```python
from build123d import *

# Parameters (mm, degrees)
SKETCH_W             = 55.4
SKETCH_H             = 49
PAD_DEPTH            = 24.5
SKETCH001_W          = 20.2
SKETCH001_H          = 39
POCKET_DEPTH         = 49
SKETCH002_W          = 20.2
SKETCH002_H          = 39
POCKET001_DEPTH      = 24.501
POCKET001_DEPTH_BACK = 24.501
SKETCH003_R          = 12.5
POCKET002_DEPTH      = 27.701
POCKET002_DEPTH_BACK = 27.701
CHAMFER_SIZE         = 1


with BuildPart() as part:
    # Sketch → Pad (new body, symmetric)
    with BuildSketch(Plane.XY):
        Rectangle(SKETCH_W, SKETCH_H)
    extrude(amount=PAD_DEPTH, both=True)

    # Sketch001 → Pocket (cut)
    with BuildSketch(Plane.XY.offset(29.5)):
        with Locations((12.6, 0)):
            Rectangle(SKETCH001_W, SKETCH001_H)
    extrude(amount=-POCKET_DEPTH, mode=Mode.SUBTRACT)

    # Sketch002 → Pocket001 (cut, two sides)
    with BuildSketch(Plane.XZ) as pocket001_sk:
        with Locations((-12.6, 0)):
            Rectangle(SKETCH002_W, SKETCH002_H)
    extrude(amount=-POCKET001_DEPTH, mode=Mode.SUBTRACT)
    extrude(pocket001_sk.sketch, amount=POCKET001_DEPTH_BACK, mode=Mode.SUBTRACT)

    # Sketch003 → Pocket002 (cut, two sides)
    with BuildSketch(Plane.YZ) as pocket002_sk:
        Circle(SKETCH003_R)
    extrude(amount=-POCKET002_DEPTH, mode=Mode.SUBTRACT)
    extrude(pocket002_sk.sketch, amount=POCKET002_DEPTH_BACK, mode=Mode.SUBTRACT)

    # Chamfer
    chamfer_edges = [part.edges().sort_by_distance(p)[0] for p in [
        (0, -24.5, 24.5),
        (-27.7, -24.5, 0),
        (0, -24.5, -24.5),
        (-12.6, -24.5, -19.5),
        (-22.7, -24.5, 0),
        (-12.6, -24.5, 19.5),
        (-2.5, -24.5, 0),
        (27.7, -24.5, 0),
        (27.7, 0, 24.5),
        (27.7, -12.5, 0),
        (27.7, 0, -24.5),
        (27.7, 24.5, 0),
        (22.7, 0, 24.5),
        (12.6, -19.5, 24.5),
        (2.5, 0, 24.5),
        (12.6, 19.5, 24.5),
        (-27.7, 0, 24.5),
        (0, 24.5, 24.5),
        (2.5, -12.5, 0),
        (22.7, -12.5, 0),
        (0, 24.5, -24.5),
        (-2.5, 24.5, 0),
        (-12.6, 24.5, -19.5),
        (-22.7, 24.5, 0),
        (-12.6, 24.5, 19.5),
        (-27.7, 24.5, 0),
        (-27.7, 0, -24.5),
        (-27.7, -12.5, 0),
        (-22.7, -12.5, 0),
        (-2.5, -12.5, 0),
    ]]
    chamfer(chamfer_edges, length=CHAMFER_SIZE)


solid = part.part
```
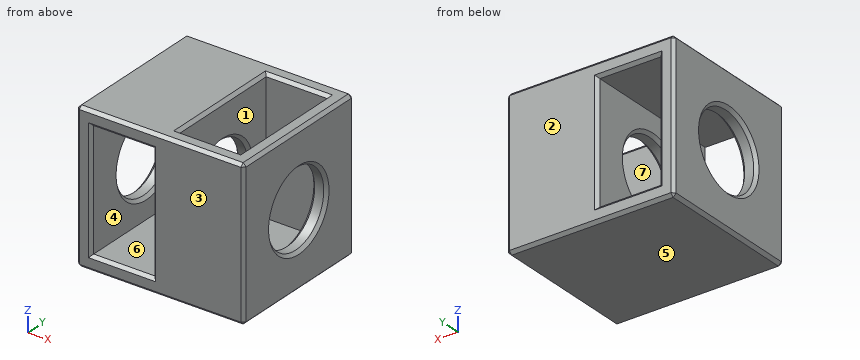
Geometry: final body of the model. Coordinates: model frame, mm. Face numbers are marked on the shaded views. A direction names the side the tool comes from. Coordinates: 2 decimals unless noted, no trailing zeros. Write each loop counter-clockwise with the first axis right and the second up, starting at its lowest first coordinate (ties: lowest second). Pieces come first, ordered by that corner, then holes. Notation, with made-up numbers: M 38,25.25 L 64,25.25 A16 ccw 64,36.25 Z; hole C -30,33.25 d6. An arc over 180 degrees is marked long. Use CSV: the item, a comma, the result in double quotes. Start each with the question number.
1. Cut plane A-A on y = -15.5. Return the cut outline in (x, z), plus the area to 4 significant figures.
2. Cut plane C-C on x = 9.5. Return the cut outline in (y, z).
3. Cut plane B-B on x = -11. Return the cut outline in (y, z), plus the area to 3 significant figures.
4. Ray query, probe 1 along X at (y, z) = (12, 9); probe 2 along Y at (x, z) = (0.5, 0); probe 3 along Y at (x, z) = (16.5, 13). Return the intervals inside material, ascending.
5. Mould query, pull axis Y, two halves, no side actions, for the marked faces 1, 2, 3 and 4. Classes: pulls with the +Y half, pulls with the -Y half, needs draft (parallel to the pull), parting line crosses it, or undercut.
6. Reachability of the marked faces 5, 6 and 7 from +Z, -Z, +X, -X, +Y, -Y: full face, straight path, thin tool, end or side. Return the list, or none.
7. Cut plane D-D on y = 0. Count the separate pieces of the cut face and the enclosed holes in it, plus the area to 3 significant figures.
8. First-contact query: P1, Ø10, axis at x = -12.5, z = 12, coming from the -Y side; P2, Ø6, axis at x = 9.5, y = 9.5, coming from the +Z side. Flat tips, straight axial feed; report the tip coordinate or a pass-through.
Entries:
1,outline,"M -27.7,-23.5 L -26.7,-24.5 L 26.7,-24.5 L 27.7,-23.5 L 27.7,23.5 L 26.7,24.5 L 23.7,24.5 L 22.7,23.5 L 22.7,-19.5 L 2.5,-19.5 L 2.5,23.5 L 1.5,24.5 L -26.7,24.5 L -27.7,23.5 Z; hole M -22.7,-19.5 L -2.5,-19.5 L -2.5,19.5 L -22.7,19.5 Z"
1,area,"1,035 mm²"
2,outline,"M -24.5,-23.5 L -23.5,-24.5 L 23.5,-24.5 L 24.5,-23.5 L 24.5,23.5 L 23.5,24.5 L 20.5,24.5 L 19.5,23.5 L 19.5,-19.5 L -19.5,-19.5 L -19.5,23.5 L -20.5,24.5 L -23.5,24.5 L -24.5,23.5 Z"
3,outline,"M -24.5,-23.5 L -23.5,-24.5 L 23.5,-24.5 L 24.5,-23.5 L 24.5,-20.5 L 23.5,-19.5 L -23.5,-19.5 L -24.5,-20.5 Z; M -24.5,20.5 L -23.5,19.5 L 23.5,19.5 L 24.5,20.5 L 24.5,23.5 L 23.5,24.5 L -23.5,24.5 L -24.5,23.5 Z"
3,area,"486 mm²"
4,probe 1,"-27.7 to -22.7, -2.5 to 2.5, 22.7 to 27.7"
4,probe 2,"-24.5 to -12.5, 12.5 to 24.5"
4,probe 3,"-24.5 to -19.5, 19.5 to 24.5"
5,face 1,"undercut"
5,face 2,"pulls with the +Y half"
5,face 3,"pulls with the -Y half"
5,face 4,"needs draft"
6,face 5,"-Z, +X, -X, +Y, -Y"
6,face 6,"+Y, -Y"
6,face 7,"+Z"
7,separate pieces,"3"
7,enclosed holes,"0"
7,area,"654 mm²"
8,P1,"through"
8,P2,"z = -19.5"
